Work out the finished part from the listing and answer in its coordinate system (mm). Face numbers are marked on the shaded views. A direction names the side the tool comes from. Coordinates: 2 decimals unless noted, no trailing zeros. Loops run counter-clockwise (first coordinate to the right, second up) from the corner with the lowest first, then second, coordinate; pieces in that order, holes last. Notation, with made-up numbers: (9, 7) -> (47, 7) arc R20 cw to (47, 37) -> close; hole circle Ø6 at (54, 20.5). An arc over 180 degrees is marked (long way). Use a Markdown table: item, result. Add a question column.
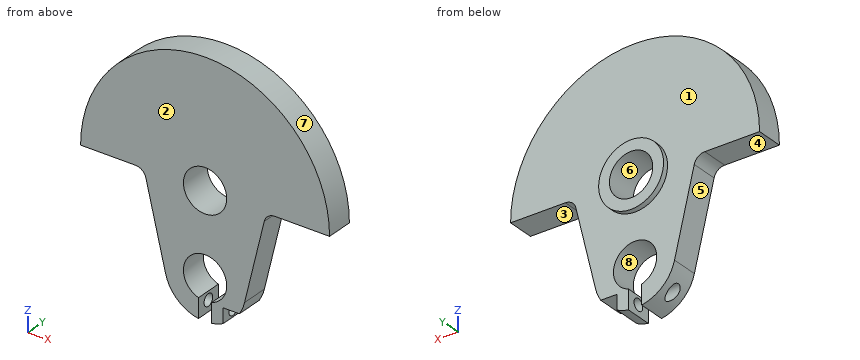
```python
from build123d import *

# Parameters (mm, degrees)
BOSS_EXTRUDE1_DEPTH     = 5
SKETCH2_R               = 6
BOSS_EXTRUDE2_DEPTH     = 1
SKETCH3_R               = 4
CUT_EXTRUDE1_DEPTH      = 34.075670817
CUT_EXTRUDE2_START      = -10
CUT_EXTRUDE2_DEPTH      = 10
CUT_EXTRUDE3_START      = -10
CUT_EXTRUDE3_DEPTH      = 10
CUT_EXTRUDE4_DEPTH      = 34.075670817
CUT_EXTRUDE4_DEPTH_BACK = 34.075670817
SKETCH7_R               = 1.0922


with BuildPart() as part:
    # Sketch1 → Boss-Extrude1 (new body)
    with BuildSketch(Plane(origin=(0, 0, 0), x_dir=(1, 0, 0), z_dir=(0, 1, 0))):
        with BuildLine():
            Line((-23, 0), (-12.87798214, 0))
            ThreePointArc((-12.87798214, 0), (-11.639160434, 0.429865999), (-10.932866059, 1.534679219))
            Line((-10.932866059, 1.534679219), (-7.294185306, 16.74495293))
            ThreePointArc((-7.294185306, 16.74495293), (0, 22.5), (7.294185306, 16.74495293))
            Line((7.294185306, 16.74495293), (10.932866059, 1.534679219))
            ThreePointArc((10.932866059, 1.534679219), (11.639160434, 0.429865999), (12.87798214, 0))
            Line((12.87798214, 0), (23, 0))
            ThreePointArc((23, 0), (0, -23), (-23, 0))
        make_face()
    extrude(amount=BOSS_EXTRUDE1_DEPTH)

    # Sketch2 → Boss-Extrude2 (add)
    with BuildSketch(Plane(origin=(0, 5, 0), x_dir=(1, 0, 0), z_dir=(0, 1, 0))):
        with Locations(Location((0, 0, 0), (0, 0, 90))):
            Circle(SKETCH2_R)
    extrude(amount=BOSS_EXTRUDE2_DEPTH)

    # Sketch3 → Cut-Extrude1 (cut, through all)
    with BuildSketch(Plane(origin=(0, 6, 0), x_dir=(1, 0, 0), z_dir=(0, 1, 0))):
        with Locations(Location((0, 0, 0), (0, 0, 270))):
            Circle(SKETCH3_R)
    extrude(amount=-CUT_EXTRUDE1_DEPTH, mode=Mode.SUBTRACT)

    # Sketch4 → Cut-Extrude2 (cut)
    with BuildSketch(Plane(origin=(0, 5, 0), x_dir=(1, 0, 0), z_dir=(0, 1, 0)).offset(CUT_EXTRUDE2_START)):
        with BuildLine():
            Line((-1.220655562, 18.809199391), (-1.220655562, 22.4))
            ThreePointArc((-1.220655562, 22.4), (0, 22.5), (1.220655562, 22.4))
            Line((1.220655562, 22.4), (1.220655562, 18.809199391))
            ThreePointArc((1.220655562, 18.809199391), (0, 11), (-1.220655562, 18.809199391))
        make_face()
    extrude(amount=CUT_EXTRUDE2_DEPTH, mode=Mode.SUBTRACT)

    # Sketch5 → Cut-Extrude3 (cut)
    with BuildSketch(Plane(origin=(0, 5, 0), x_dir=(1, 0, 0), z_dir=(0, 1, 0)).offset(CUT_EXTRUDE3_START)):
        with BuildLine():
            Line((3.34428877, 19), (6.34428877, 19))
            ThreePointArc((6.34428877, 19), (5.030642475, 20.562610564), (3.34428877, 21.713101565))
            Line((3.34428877, 21.713101565), (3.34428877, 19))
        make_face()
    extrude(amount=CUT_EXTRUDE3_DEPTH, mode=Mode.SUBTRACT)

    # Sketch7 → Cut-Extrude4 (cut, two sides: drawn at the far end of the back side and taken through both)
    with BuildSketch(Plane(origin=(0, 0, 0), x_dir=(0, 0, -1), z_dir=(1, 0, 0)).offset(-CUT_EXTRUDE4_DEPTH_BACK)):
        with Locations((20.358101565, 2.5)):
            Circle(SKETCH7_R)
    extrude(amount=CUT_EXTRUDE4_DEPTH + CUT_EXTRUDE4_DEPTH_BACK, mode=Mode.SUBTRACT)


solid = part.part
```
Item 1: Section A-A (x = 0) is taken. Determine the outline of the cut face in (y, z), then the cut area to 3 significant figures.
Item 2: Section C-C (z = -15) is taken. Determine the outline of the cut face in (x, y).
Item 3: Find the intervals of material crossed by probe 1 along Z at (x, y) = (2.15, 2.5); probe 2 along Y at (x, z) = (-10.5, -3); probe 3 along Z at (x, y) = (-3.2, 2.5), in increasing order.
Item 4: Section D-D (z = -5) is taken. Determine the outline of the cut face in (x, y).
Item 5: For a pull along Z with two mould halves and no side action, classify the marked faces 5, 6, 7 and 8 as +Z half, -Z half, draft (parallel to the pull), parting line (faces both ways), or undercut.
Item 6: For the marked faces 1, 2, 3 and 4, determine the directions among +Z, -Z, +X, -X, +Y, -Y from which every point of the face is accessible in a straight line to the end or side of a thin tool.
Item 7: Section B-B (y = 2.5) is taken. Determine the outline of the cut face in (x, z), then the cut area to 3 significant figures.
Item 8: Given pin 1 (1 mm diameter, centred on x = -16.5, z = 15.5, fed in from +Y); pin 2 (2.5 mm diameter, centred on x = -16, y = 1.5, fed in from -Z); pin 3 (2 mm diameter, centred on y = 3, z = -20.5, fed in from +X), each flat-ended and moving along its own axis, determine where each tip first touches the part or whether it passes through.
Output:
| question | item | result |
|---|---|---|
| 1 | outline | (0, -11) -> (5, -11) -> (5, -6) -> (6, -6) -> (6, -4) -> (0, -4) -> close; (0, 4) -> (6, 4) -> (6, 6) -> (5, 6) -> (5, 23) -> (0, 23) -> close |
| 1 | area | 134 mm2 |
| 2 | outline | (-7.71, 0) -> (-4, 0) -> (-4, 5) -> (-7.71, 5) -> close; (4, 0) -> (7.71, 0) -> (7.71, 5) -> (4, 5) -> close |
| 3 | probe 1 | z = -22.19 to -21.45, -19.27 to -18.37, -11.63 to -3.37, 3.37 to 22.9 |
| 3 | probe 2 | y = 0 to 5 |
| 3 | probe 3 | z = -21.78 to -21.45, -19.27 to -17.4, -12.6 to -2.4, 2.4 to 22.78 |
| 4 | outline | (-10.1, 0) -> (10.1, 0) -> (10.1, 5) -> (3.32, 5) -> (3.32, 6) -> (-3.32, 6) -> (-3.32, 5) -> (-10.1, 5) -> close |
| 5 | face 5 | -Z half |
| 5 | face 6 | undercut |
| 5 | face 7 | +Z half |
| 5 | face 8 | undercut |
| 6 | face 1 | +Y |
| 6 | face 2 | +Z, -Z, +X, -X, -Y |
| 6 | face 3 | -Z, +X, +Y, -Y |
| 6 | face 4 | -Z, -X, +Y, -Y |
| 7 | outline | (-23, 0) -> (-12.88, 0) arc R2 cw to (-10.93, -1.53) -> (-7.29, -16.74) arc R7.5 ccw to (-6.17, -19.27) -> (-1.22, -19.27) -> (-1.22, -18.81) arc R4 cw (long way) to (1.22, -18.81) -> (1.22, -19.27) -> (3.34, -19.27) -> (3.34, -19) -> (6.34, -19) arc R7.5 ccw to (7.29, -16.74) -> (10.93, -1.53) arc R2 cw to (12.88, 0) -> (23, 0) arc R23 ccw to start; (-3.83, -21.45) arc R7.5 ccw to (-1.22, -22.4) -> (-1.22, -21.45) -> close; (1.22, -22.4) arc R7.5 ccw to (3.34, -21.71) -> (3.34, -21.45) -> (1.22, -21.45) -> close; hole circle Ø8 at (0, 0) |
| 7 | area | 1,080 mm2 |
| 8 | pin 1 | stops at y = 5 |
| 8 | pin 2 | stops at z = 0 |
| 8 | pin 3 | stops at x = 3.34 |
